The listing builds one solid part. Answer for the finished solid, in the listing's coordinates (mm). A direction names the side the tool comes from. Give positions to 0.01 mm unless a question says otherwise; leave off trailing zeros. Write each loop counter-clockwise with the first axis right and the second up, starting at its lowest first coordinate (ties: lowest second). Pieces come first, ordered by that corner, then holes. Notation, with made-up numbers: (33, -15.75) - (48, -15.75) arc R22 cw to (48, -1.75) - close; hole circle Ø7 at (27.25, 82). An arc over 180 degrees is marked (long way). Answer in a Markdown table with one row per item. Add a question column.
from build123d import *

# Parameters (mm, degrees)
F1_DEPTH = 508


with BuildPart() as f1:
    # F0 (on Top) → F1 (new body)
    with BuildSketch(Plane.XY):
        with BuildLine():
            Line((168.20993, 223.271681), (-161.99007, 223.271681))
            Line((-161.99007, 223.271681), (-161.99007, -58.067597))
            Line((-161.99007, -58.067597), (-161.99007, -66.242225))
            ThreePointArc((-161.99007, -66.242225), (-113.341942, -179.388298), (0, -227.578319))
            Line((0, -227.578319), (6.836314, -227.578319))
            ThreePointArc((6.836314, -227.578319), (116.300399, -183.126755), (168.20993, -76.996043))
            Line((168.20993, -76.996043), (168.20993, -47.313779))
            Line((168.20993, -47.313779), (168.20993, 223.271681))
        make_face()
        with BuildLine():
            Line((-161.99007, -66.242225), (-161.99007, -58.067597))
            ThreePointArc((-161.99007, -58.067597), (-162.040562, -62.154911), (-161.99007, -66.242225))
        make_face()
        with BuildLine():
            ThreePointArc((168.20993, -76.996043), (168.876876, -62.154911), (168.20993, -47.313779))
            Line((168.20993, -47.313779), (168.20993, -76.996043))
        make_face()
        with BuildLine():
            Line((6.836314, -227.578319), (0, -227.578319))
            ThreePointArc((0, -227.578319), (3.418157, -227.61363), (6.836314, -227.578319))
        make_face()
    extrude(amount=F1_DEPTH)


solid = f1.part
1. A tool of negligible diameter and unlimited length cuts with its end or side. For faces 1 (the face through (168.877, -62.363, 250.444)), 2 (the face through (168.21, 86, 250)), from which of +Z, -Z, +X, -X, +Y, -Y can it reach the whole face along a straight path? Write none if from no direction.
2. Section B-B (y = -143.5) is taken. Give the vertices of the cut face in (x, z), and give its area (3 significant figures).
3. Section C-C (x = -105) is taken. Give the vertices of the cut face in (y, z), and give its area (3 significant figures).
4. Straight lines are drawn through the part: L1, parallel to X at y = 10, z = 100.5; L2, parallel to Y at x = 5, z = 222; L3, parallel to X at y = -55.5, z = 294. For each, find the intervals that lie inside material, in ascending order. Write a range as [from, to].
5. Given pin 1 Ø6 at (x, z) = (-112, 165) entering from -Y; pin 2 Ø12 at (x, z) = (-46, 392.5) entering from -Y; pin 3 Ø2 at (x, z) = (-48.5, 187) entering from -Y, each flat-ended and moving along its own axis, determine where each tip first touches the part or whether it passes through.
6. Section A-A (z = 359) is taken. Give the vertices of the cut face in (x, y).
Geometry check:
| question | item | result |
|---|---|---|
| 1 | face 1 | +Z, -Z, +X |
| 1 | face 2 | +Z, -Z, +X, +Y |
| 2 | outline | (-140.66, 0) - (147.5, 0) - (147.5, 508) - (-140.66, 508) - close |
| 2 | area | 146,000 mm² |
| 3 | outline | (-187.14, 0) - (223.27, 0) - (223.27, 508) - (-187.14, 508) - close |
| 3 | area | 208,000 mm² |
| 4 | L1 | [-161.99, 168.21] |
| 4 | L2 | [-227.61, 223.27] |
| 4 | L3 | [-161.99, 168.74] |
| 5 | pin 1 | y = -183.56 |
| 5 | pin 2 | y = -221.82 |
| 5 | pin 3 | y = -219.58 |
| 6 | outline | (-161.99, -66.24) arc R165.46 ccw to (0, -227.58) arc R165.46 ccw to (6.84, -227.58) arc R165.46 ccw to (168.21, -77) arc R165.46 ccw to (168.21, -47.31) - (168.21, 223.27) - (-161.99, 223.27) - (-161.99, -58.07) arc R165.46 ccw to start |
